Can you work these out from the drawing? Everything is in mm from the part's minimum corner. Round coordinates to 2 decimals unless told otherwise and drop trailing zeros. Order: outer loops, then holes, each group sorted by start corner. A loop starts at its lowest first (then second) coordinate and runs counter-clockwise, first axis right, second up. Notation, with made-up numbers: (40, -2.5) - (82, -2.5) arc R11 cw to (82, 11.5) - close; hole circle Ø2 at (34.5, 27). An arc over 180 degrees is marked (long way). Write item = value, one per line.
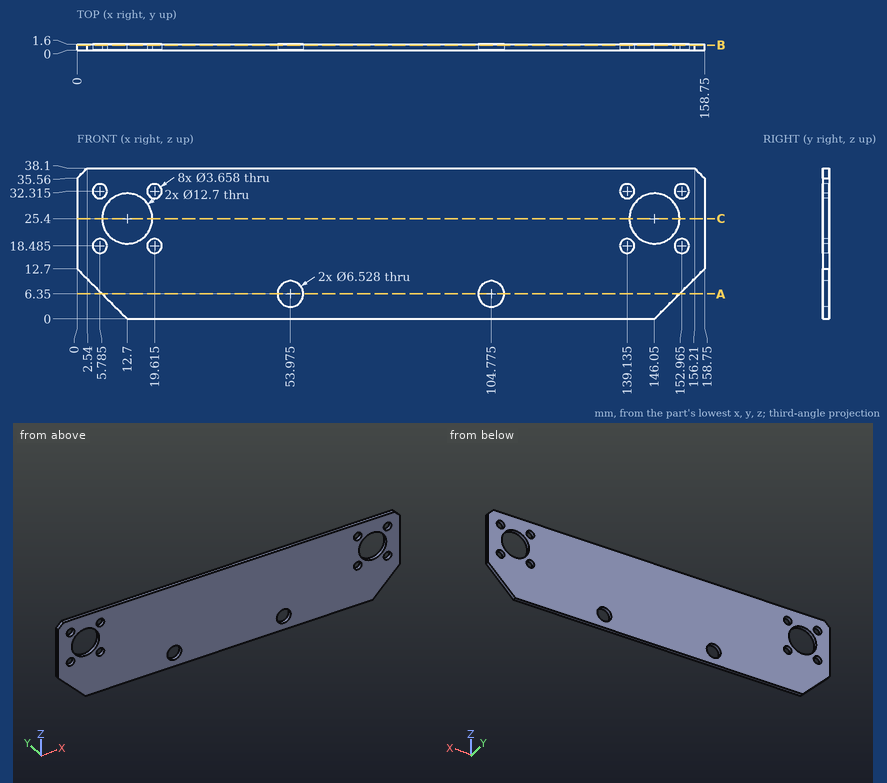
(1) If I drill on line 1 (Z direction, x = 12.7, y = 0.8); line 2 (X direction, y = 0.9, z = 21.5); line 3 (X direction, y = 0.6, z = 29.5), over which ranges is the centre line in solid material (lowest first)? Write a range as from..to.
Computed:
line_1 = 0..19.05, 31.75..38.1
line_2 = 0..7.69, 17.71..141.04, 151.06..158.75
line_3 = 0..7.85, 17.55..141.2, 150.9..158.75
(2) Will these pins go through, and if not, where does the flat tip stop? P1, Ø4, axis at x = 139.14, z = 32.31, coming from the -Y side; P2, Ø7.5, axis at x = 12.7, z = 25.4, coming from the +Y side.
Computed:
P1 = 0
P2 = through
(3) If we section it at A-A (z = 6.35): Write out the boundary of the cut face in (x, y).
Computed:
outline = (6.35, 0) - (50.71, 0) - (50.71, 1.6) - (6.35, 1.6) - close; (57.24, 0) - (101.51, 0) - (101.51, 1.6) - (57.24, 1.6) - close; (108.04, 0) - (152.4, 0) - (152.4, 1.6) - (108.04, 1.6) - close
(4) If we section it at C-C (z = 25.4): Write out the boundary of the cut face in (x, y).
Computed:
outline = (0, 0) - (6.35, 0) - (6.35, 1.6) - (0, 1.6) - close; (19.05, 0) - (139.7, 0) - (139.7, 1.6) - (19.05, 1.6) - close; (152.4, 0) - (158.75, 0) - (158.75, 1.6) - (152.4, 1.6) - close
(5) If we section it at B-B (y = 1.3): State how many separate pieces and enclosed holes the cut face has, plus the area to 3 significant figures.
Computed:
separate_pieces = 1
enclosed_holes = 12
area = 5,480 mm^2
